The listing builds one solid part. Answer for the finished solid, in the listing's coordinates (mm). Face numbers are marked on the shaded views. A direction names the side the tool comes from. Coordinates: 2 decimals unless noted, no trailing zeros. Order: outer loops, then holes, each group sorted by start corner. A loop starts at its lowest first (then second) coordinate and runs counter-clockwise, first axis right, second up. Notation, with made-up numbers: (23, 30.25) -> (35, 30.25) arc R17 ccw to (35, 42.25) -> close; hole circle Ø1 at (67, 69.25). An arc over 180 degrees is marked (long way). Return JSON: item names as keys, results as strings.
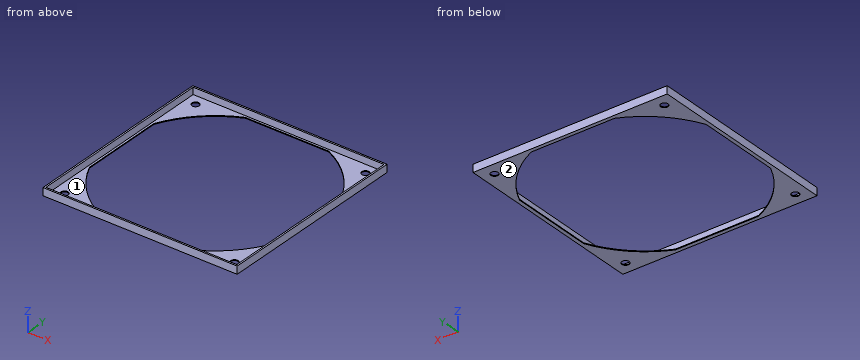
from build123d import *

# Parameters (mm, degrees)
F1_W     = 142.4
F1_H     = 142.4
F4_DEPTH = 0.6
F2_W     = 142.4
F2_H     = 142.4
F2_W_2   = 140
F2_H_2   = 140
F5_DEPTH = 5
F3_R     = 2.7
F6_DEPTH = 0.601


with BuildPart() as f4:
    # F1 (on Top) → F4 (new body)
    with BuildSketch(Plane.XY):
        Rectangle(F1_W, F1_H)
        with BuildLine():
            ThreePointArc((-68.5, 30.540956), (-53.033009, 53.033009), (-30.540956, 68.5))
            Line((-30.540956, 68.5), (30.540956, 68.5))
            ThreePointArc((30.540956, 68.5), (53.033009, 53.033009), (68.5, 30.540956))
            Line((68.5, 30.540956), (68.5, -30.540956))
            ThreePointArc((68.5, -30.540956), (53.033009, -53.033009), (30.540956, -68.5))
            Line((30.540956, -68.5), (-30.540956, -68.5))
            ThreePointArc((-30.540956, -68.5), (-53.033009, -53.033009), (-68.5, -30.540956))
            Line((-68.5, -30.540956), (-68.5, 30.540956))
        make_face(mode=Mode.SUBTRACT)
    extrude(amount=-F4_DEPTH)

    # F2 (on Top) → F5 (join)
    with BuildSketch(Plane.XY):
        Rectangle(F2_W, F2_H)
        Rectangle(F2_W_2, F2_H_2, mode=Mode.SUBTRACT)
    extrude(amount=F5_DEPTH)

    # F3 (on Top) → F6 (cut, through all)
    with BuildSketch(Plane.XY):
        with Locations((62.25, 62.25)):
            Circle(F3_R)
        with Locations((-62.25, 62.25)):
            Circle(F3_R)
        with Locations((-62.25, -62.25)):
            Circle(F3_R)
        with Locations((62.25, -62.25)):
            Circle(F3_R)
    extrude(amount=-F6_DEPTH, mode=Mode.SUBTRACT)


solid = f4.part
1. Consider line 1 (X direction, y = 52.5, z = 4.85); line 2 (X direction, y = 12, z = -0.3). Determine where each line is inside the solid, lowest interval first. Write a range as from..to.
Answer block:
{"line 1": "x = -71.2..-70, 70..71.2", "line 2": "x = -71.2..-68.5, 68.5..71.2"}
2. The part is cut by section C-C on z = 2.7. Give the vertices of the cut face in (x, y).
Answer block:
{"outline": "(-71.2, -71.2) -> (71.2, -71.2) -> (71.2, 71.2) -> (-71.2, 71.2) -> close; hole (-70, -70) -> (70, -70) -> (70, 70) -> (-70, 70) -> close"}
3. The part is cut by section A-A on x = -23.5. Give the vertices of the cut face in (y, z), and give its area (3 significant figures).
Answer block:
{"outline": "(-71.2, -0.6) -> (-68.5, -0.6) -> (-68.5, 0) -> (-70, 0) -> (-70, 5) -> (-71.2, 5) -> close; (68.5, -0.6) -> (71.2, -0.6) -> (71.2, 5) -> (70, 5) -> (70, 0) -> (68.5, 0) -> close", "area": "15.2 mm2"}
4. Each of these flat-tipped pins is pushed along its axis until it touches: pin 1 Ø8.5 at (x, y) = (-62.25, -62.25) entering from +Z; pin 2 Ø6 at (x, y) = (62.25, -62.25) entering from -Z. Where does it stop, or does it pass through?
Answer block:
{"pin 1": "stops at z = 0", "pin 2": "stops at z = -0.6"}
5. The part is cut by section D-D on x = -62.25. Give the vertices of the cut face in (y, z), and give its area (3 significant figures).
Answer block:
{"outline": "(-71.2, -0.6) -> (-64.95, -0.6) -> (-64.95, 0) -> (-70, 0) -> (-70, 5) -> (-71.2, 5) -> close; (-59.55, -0.6) -> (-41.83, -0.6) -> (-41.83, 0) -> (-59.55, 0) -> close; (41.83, -0.6) -> (59.55, -0.6) -> (59.55, 0) -> (41.83, 0) -> close; (64.95, -0.6) -> (71.2, -0.6) -> (71.2, 5) -> (70, 5) -> (70, 0) -> (64.95, 0) -> close", "area": "40.8 mm2"}
6. For the marked faces 1 and 2, determine the directions among +Z, -Z, +X, -X, +Y, -Y from which every point of the face is accessible in a straight line to the end or side of a thin tool.
Answer block:
{"face 1": "+Z", "face 2": "-Z, +X, -X, +Y, -Y"}
